Autodesk Inventor part; units mm, degrees
ref_plane "YZ Plane" through (0, 0, 0) normal (1, 0, 0) x (0, 1, 0)
ref_plane "XZ Plane" through (0, 0, 0) normal (0, 1, 0) x (-1, 0, 0)
ref_plane "XY Plane" through (0, 0, 0) normal (0, 0, 1) x (1, 0, 0)
sketch "Sketch1" plane through (0, 0, 0) normal (0, 1, 0) x (-1, 0, 0)
  line L0 (1, 0) -> (58, 0)
  line L1 (59, -1) -> (59, -71)
  line L2 (58, -72) -> (1, -72)
  line L3 (0, -71) -> (0, -1)
  arc A0 (59, -1) -> (58, 0) centre (58, -1) ccw
  arc A1 (58, -72) -> (59, -71) centre (58, -71) ccw
  arc A2 (0, -71) -> (1, -72) centre (1, -71) ccw
  arc A3 (1, 0) -> (0, -1) centre (1, -1) ccw
  point P0 (0, 0)
  point P1 (59, -72)
  point P2 (59, 0)
  point P3 (0, -72)
  dimension "d0" = 72
  dimension "d1" = 59
  dimension "d2" = 1
extrude "Extrusion1" add sketch "Sketch1" along normal blind 1
sketch "Sketch2" plane through (0, 1, 0) normal (0, 1, 0) x (1, 0, 0)
  line L0 (-55.9113, 2.4272) -> (-2.9113, 2.4272)
  line L1 (-2.9113, 2.4272) -> (-2.9113, 32.4272)
  line L2 (-2.9113, 32.4272) -> (-55.9113, 32.4272)
  line L3 (-55.9113, 32.4272) -> (-55.9113, 2.4272)
  line L4 (-56.4113, 1.9272) -> (-2.4113, 1.9272)
  line L5 (-2.4113, 1.9272) -> (-2.4113, 32.9272)
  line L6 (-2.4113, 32.9272) -> (-56.4113, 32.9272)
  line L7 (-56.4113, 32.9272) -> (-56.4113, 1.9272)
  point P0 (0, 0)
  dimension "d5" = 30
  dimension "d6" = 53
  dimension "d7" = 0.5
  dimension "d8" = 0.5
  dimension "d9" = 0.5
  dimension "d10" = 0.5
extrude "Extrusion2" add sketch "Sketch2" along normal blind 4
sketch "Sketch3" plane through (0, 1, 0) normal (0, 1, 0) x (1, 0, 0)
  arc A0 (0, 71) -> (-1, 72) centre (-1, 71) ccw
  line L0 (-58, 1) -> (-1, 1)
  line L1 (-1, 1) -> (-1, 71)
  line L2 (-1, 71) -> (-58, 71)
  line L3 (-58, 71) -> (-58, 1)
  line L4 (-1, 72) -> (-58, 72)
  line L5 (-59, 71) -> (-59, 1)
  line L6 (-58, 0) -> (-1, 0)
  line L7 (0, 1) -> (0, 71)
  point P0 (0, 0)
  dimension "d13" = 1
  dimension "d14" = 1
  dimension "d15" = 1
  dimension "d16" = 1
extrude "Extrusion3" add sketch "Sketch3" along normal blind 1
sketch "Sketch4" plane through (0, 5, 0) normal (0, 1, 0) x (1, 0, 0)
  line L0 (-2.4113, 1.9272) -> (-2.4113, 32.9272)
  line L1 (-2.9113, 32.4272) -> (-2.9113, 2.4272)
  line L2 (-56.4113, 1.9272) -> (-2.4113, 1.9272)
  line L3 (-2.9113, 2.4272) -> (-55.9113, 2.4272)
  line L4 (-2.4113, 32.9272) -> (-56.4113, 32.9272)
  line L5 (-55.9113, 32.4272) -> (-2.9113, 32.4272)
  line L6 (-55.9113, 2.4272) -> (-55.9113, 32.4272)
  line L7 (-56.4113, 32.9272) -> (-56.4113, 1.9272)
  point P0 (0, 0)
extrude "Extrusion4" add sketch "Sketch4" along normal blind 5
sketch "Sketch5" plane through (-2.4113, 2, -1.9272) normal (1, 0, 0) x (0, 0, -1)
  line L0 (0, 0) -> (31, 0)
  line L1 (31, 0) -> (31, 8)
  line L2 (0, 8) -> (31, 8)
  line L3 (0, 0) -> (0, 8)
  circle A0 centre (15.5, 4) radius 2
  point P0 (-1.9272, -2)
  dimension "d21" = 4
extrude "Extrusion6" cut sketch "Sketch5" against normal through all contours A0
sketch "Sketch7" plane through (-2.4113, 2, -32.9272) normal (0, 0, -1) x (-1, 0, 0)
  line L0 (0, 0) -> (54, 0)
  line L1 (54, 0) -> (54, 8)
  line L2 (0, 8) -> (54, 8)
  line L3 (0, 0) -> (0, 8)
  circle A0 centre (27, 4) radius 1.5
  point P0 (-2.4113, -2)
  dimension "d26" = 3
extrude "Extrusion7" cut sketch "Sketch7" against normal blind 3 contours A0
properties part number "tapa caja arduino"
Source: CAD feature listing. Evaluate the final solid. Frame: model axes, mm. A direction names the side the tool comes from. Round coordinates to 2 decimals unless told otherwise and drop trailing zeros. Loops run counter-clockwise (first coordinate to the right, second up) from the corner with the lowest first, then second, coordinate; pieces in that order, holes last.
(1) Material intervals for probe 1 along X at (y, z) = (9.5, -11); probe 2 along Z at (x, y) = (-27, 6); probe 3 along Y at (x, z) = (-36, -56), sorted ascending.
From the geometry:
probe 1: x = -56.41 to -55.91, -2.91 to -2.41
probe 2: z = -32.93 to -32.43, -2.43 to -1.93
probe 3: y = 0 to 2
(2) Contact query for flat-ended pins moving along their axis: pin 1 Ø2.5 at (x, y) = (-28, 7) entering from +Z; pin 2 Ø17.5 at (x, z) = (-43.5, -47) entering from +Y; pin 3 Ø4.5 at (y, z) = (6, -17.43) entering from +X. Output: stop coordinate, or through.
From the geometry:
pin 1: stops at z = -1.93
pin 2: stops at y = 2
pin 3: stops at x = -2.41
(3) Section query A-A (y = 9.25). Output: boundary loops of the cut face in (x, z), and give its area (3 significant figures).
From the geometry:
outline: (-56.41, -32.93) - (-2.41, -32.93) - (-2.41, -1.93) - (-56.41, -1.93) - close; hole (-55.91, -32.43) - (-2.91, -32.43) - (-2.91, -2.43) - (-55.91, -2.43) - close
area: 84.0 mm2
(4) Section query B-B (x = -40.5). Output: boundary loops of the cut face in (y, z), and give its area (3 significant figures).
From the geometry:
outline: (0, -72) - (1, -72) - (1, -71) - (2, -71) - (2, -32.93) - (10, -32.93) - (10, -32.43) - (2, -32.43) - (2, -2.43) - (10, -2.43) - (10, -1.93) - (2, -1.93) - (2, -1) - (1, -1) - (1, 0) - (0, 0) - close
area: 150 mm2
(5) Section query C-C (z = -59). Output: boundary loops of the cut face in (x, y).
From the geometry:
outline: (-59, 0) - (0, 0) - (0, 1) - (-1, 1) - (-1, 2) - (-58, 2) - (-58, 1) - (-59, 1) - close
(6) Access query for faces 1 (the flat face through (-29, 4, -32.927)), 2 (the flat face through (-55.911, 3, -17)), 3 (the flat face through (-56.411, 3, -18)), 4 (the flat face through (-2.411, 3, -17)), 5 (the cylindrical face through (-30.842, 6.451, -32.681)). Directions: +Z, -Z, +X, -X, +Y, -Y. A direction counts if a zero-diameter tool reaches every point of the face in a straight line with its end or side. Return the directions, or none.
From the geometry:
face 1: -Z, +X, -X, +Y
face 2: +Y
face 3: +Z, -Z, -X, +Y
face 4: +Z, -Z, +X, +Y
face 5: -Z
(7) Pull-direction query (Y, two-part tool) for faces 6 (the cylindrical face through (-56.158, 6.601, -19.335)), 7 (the flat face through (-29, 0, -35)), 8 (the flat face through (-30, 4, -32.427)); classes: +Y half, -Y half, draft (parallel to the pull), parting line (faces both ways), or undercut.
From the geometry:
face 6: undercut
face 7: -Y half
face 8: draft
